from build123d import *

# Parameters (mm, degrees)
F0_R     = 3.8
F1_DEPTH = 4


# Not quite as in the source:
# - a feature names something its author has since deleted; it is built from what else it names


with BuildPart() as f1:
    # F0 (on Top) → F1 (new body)
    with BuildSketch(Plane.XY):
        with BuildLine():
            ThreePointArc((10.7032142857, -9.0244780433), (13.15, -4.8039046618), (14, 0))
            ThreePointArc((14, 0), (13.2657182303, 4.4744519031), (11.1398971667, 8.4795454545))
            ThreePointArc((11.1398971667, 8.4795454545), (-3.1423826746, 13.6427794502), (-13.7268716756, 2.7519073388))
            ThreePointArc((-13.7268716756, 2.7519073388), (-12.8265756347, -5.610611151), (-7.2967857143, -11.9480926612))
            ThreePointArc((-7.2967857143, -11.9480926612), (-3.7899012351, -13.4772641374), (0, -14))
            ThreePointArc((0, -14), (5.90158061, -12.6953277352), (10.7032142857, -9.0244780433))
        make_face()
        Circle(F0_R, mode=Mode.SUBTRACT)
        with BuildLine():
            ThreePointArc((4.0123564651, -48.3244780433), (13.6087273384, -29.7387061328), (10.7032142857, -9.0244780433))
            ThreePointArc((10.7032142857, -9.0244780433), (5.90158061, -12.6953277352), (0, -14))
            ThreePointArc((0, -14), (-3.7899012351, -13.4772641374), (-7.2967857143, -11.9480926612))
            ThreePointArc((-7.2967857143, -11.9480926612), (1.6235591613, -27.8480926612), (-7.2967857143, -43.7480926612))
            ThreePointArc((-7.2967857143, -43.7480926612), (-6.2932161351, -83.0480926612), (-7.2967857143, -122.3480926612))
            ThreePointArc((-7.2967857143, -122.3480926612), (-0.8068871669, -125.4847000324), (4.0123564651, -120.1244780433))
            ThreePointArc((4.0123564651, -120.1244780433), (5.0200325676, -84.2244780433), (4.0123564651, -48.3244780433))
        make_face()
        with BuildLine():
            ThreePointArc((-13.7268716756, 2.7519073388), (-3.1423826746, 13.6427794502), (11.1398971667, 8.4795454545))
            ThreePointArc((11.1398971667, 8.4795454545), (2.1510025477, 35.1295454545), (11.1398971667, 61.7795454545))
            ThreePointArc((11.1398971667, 61.7795454545), (11.6091204752, 64.5781543581), (9.0255790591, 65.7519073388))
            ThreePointArc((9.0255790591, 65.7519073388), (-10.5763059667, 37.2226044204), (-13.7268716756, 2.7519073388))
        make_face()
    extrude(amount=F1_DEPTH)


solid = f1.part
Input: part model. Units: mm. Frame: model coordinates. Coordinates: 2 decimals unless noted, no trailing zeros. Loops run counter-clockwise (first coordinate to the right, second up) from the corner with the lowest first, then second, coordinate; pieces in that order, holes last.
Q1. Cut plane B-B (z = 2.3). Output: boundary loops of the cut face in (x, y), then the cut area to 3 significant figures.
Q2. Material intervals for line 1 (Y direction, x = 0, z = 1.85); line 2 (Y direction, x = 11.5, z = 2.15); line 3 (Y direction, x = 6.75, z = 2), sorted ascending.
Q3. Cut plane C-C (y = -91). Output: boundary loops of the cut face in (x, z).
Q4. Draft query along Y for faces 1 (the face through (3, -29, 4)), 2 (the face through (-0.913, -125.505, 1.972)), 3 (the face through (-12.874, -5.501, 1.972)). Return one class per face: +Y half, -Y half, draft (parallel to the pull), parting line (faces both ways), or undercut.
Q5. Cut plane D-D (y = 18). Output: boundary loops of the cut face in (x, z), then the cut area to 3 significant figures.
Q6. Cut plane A-A (x = 0). Output: boundary loops of the cut face in (y, z).
Q7. Contact query for flat-ended pins moving along their axis: pin 1 (1 mm diameter, centred on x = -4.5, z = 3.5, fed in from -Y); pin 2 (1.5 mm diameter, centred on x = -10, z = 3.5, fed in from -Y). Output: stop coordinate, or through.
Working result:
1. outline: (-13.73, 2.75) arc R14 ccw to (-7.3, -11.95) arc R18.63 cw to (-7.3, -43.75) arc R770 cw to (-7.3, -122.35) arc R6 ccw to (4.01, -120.12) arc R640 ccw to (4.01, -48.32) arc R34.5 ccw to (10.7, -9.02) arc R14 ccw to (11.14, 8.48) arc R44 cw to (11.14, 61.78) arc R2.33 ccw to (9.03, 65.75) arc R68.5 ccw to start; hole circle Ø7.6 at (0, 0)
1. area: 2,600 mm2
2. line 1: y = -125.27 to -35.45, -20.24 to -3.8, 3.8 to 56.29
2. line 2: y = -37.08 to -10.81, -7.98 to 7.98, 62.21 to 64.76
2. line 3: y = -45.23 to 15.54, 54.71 to 63.69
3. outline: (-6.33, 0) - (4.98, 0) - (4.98, 4) - (-6.33, 4) - close
4. face 1: draft
4. face 2: -Y half
4. face 3: undercut
5. outline: (-14.53, 0) - (5.62, 0) - (5.62, 4) - (-14.53, 4) - close
5. area: 80.6 mm2
6. outline: (-125.27, 0) - (-35.45, 0) - (-35.45, 4) - (-125.27, 4) - close; (-20.24, 0) - (-3.8, 0) - (-3.8, 4) - (-20.24, 4) - close; (3.8, 0) - (56.29, 0) - (56.29, 4) - (3.8, 4) - close
7. pin 1: stops at y = -125.24
7. pin 2: stops at y = -10.51
